from build123d import *

# Parameters (mm, degrees)
SKETCH1_W           = 140
SKETCH1_H           = 200
BOSS_EXTRUDE1_DEPTH = 30
SKETCH2_W           = 140
SKETCH2_H           = 15
CUT_EXTRUDE1_DEPTH  = 175.642491966
SKETCH3_W           = 60
SKETCH3_H           = 15
CUT_EXTRUDE3_DEPTH  = 215.00934559
SKETCH4_W           = 80
SKETCH4_H           = 140
BOSS_EXTRUDE3_DEPTH = 61
SKETCH5_W           = 100
SKETCH5_H           = 160
SKETCH5_W_2         = 70
SKETCH5_H_2         = 130
BOSS_EXTRUDE4_DEPTH = 14
SKETCH7_W           = 70
SKETCH7_H           = 130
CUT_EXTRUDE4_DEPTH  = 36
BOSS_EXTRUDE5_DEPTH = 10
BOSS_EXTRUDE6_DEPTH = 10


with BuildPart() as part:
    # Sketch1 → Boss-Extrude1 (new body)
    with BuildSketch(Plane(origin=(0, 0, 0), x_dir=(1, 0, 0), z_dir=(0, 1, 0))):
        Rectangle(SKETCH1_W, SKETCH1_H)
    extrude(amount=BOSS_EXTRUDE1_DEPTH)

    # Sketch2 → Cut-Extrude1 (cut, through all)
    with BuildSketch(Plane(origin=(70, 0, 0), x_dir=(0, 0, -1), z_dir=(1, 0, 0))):
        with Locations((0, 7.5)):
            Rectangle(SKETCH2_W, SKETCH2_H)
    extrude(amount=-CUT_EXTRUDE1_DEPTH, mode=Mode.SUBTRACT)

    # Sketch3 → Cut-Extrude3 (cut, through all)
    with BuildSketch(Plane.XY.offset(100)):
        with Locations((0, 7.5)):
            Rectangle(SKETCH3_W, SKETCH3_H)
    extrude(amount=-CUT_EXTRUDE3_DEPTH, mode=Mode.SUBTRACT)

    # Sketch4 → Boss-Extrude3 (add)
    with BuildSketch(Plane(origin=(0, 30, 0), x_dir=(1, 0, 0), z_dir=(0, 1, 0))):
        Rectangle(SKETCH4_W, SKETCH4_H)
    extrude(amount=BOSS_EXTRUDE3_DEPTH)

    # Sketch5 → Boss-Extrude4 (add)
    with BuildSketch(Plane(origin=(0, 91, 0), x_dir=(1, 0, 0), z_dir=(0, 1, 0))):
        Rectangle(SKETCH5_W, SKETCH5_H)
        Rectangle(SKETCH5_W_2, SKETCH5_H_2, mode=Mode.SUBTRACT)
    extrude(amount=BOSS_EXTRUDE4_DEPTH)

    # Sketch7 → Cut-Extrude4 (cut)
    with BuildSketch(Plane(origin=(0, 91, 0), x_dir=(1, 0, 0), z_dir=(0, 1, 0))):
        Rectangle(SKETCH7_W, SKETCH7_H)
    extrude(amount=-CUT_EXTRUDE4_DEPTH, mode=Mode.SUBTRACT)

    # Sketch9 → Boss-Extrude5 (add, symmetric)
    with BuildSketch(Plane.XY):
        Polygon((-50, 91), (-70, 30), (-39.979727261, 30), (-40, 91), align=None)
    boss_extrude5 = extrude(amount=BOSS_EXTRUDE5_DEPTH, both=True)

    # Mirror1: Boss-Extrude5 across plane
    add(boss_extrude5.mirror(Plane(origin=(0, 0, 0), x_dir=(0, 0, 1), z_dir=(1, 0, 0))))

    # Sketch10 → Boss-Extrude6 (add, symmetric)
    with BuildSketch(Plane(origin=(0, 0, 0), x_dir=(0, 0, -1), z_dir=(1, 0, 0))):
        Polygon((-70, 91), (-80, 91), (-100, 30), (-70, 30), align=None)
    boss_extrude6 = extrude(amount=BOSS_EXTRUDE6_DEPTH, both=True)

    # Mirror2: Boss-Extrude6 across plane
    add(boss_extrude6.mirror(Plane.XY))


solid = part.part
The model under review builds one solid part; all positions refer to its coordinate system, in mm. A direction names the side the tool comes from. Round coordinates to 2 decimals unless told otherwise and drop trailing zeros. Order: outer loops, then holes, each group sorted by start corner. A loop starts at its lowest first (then second) coordinate and runs counter-clockwise, first axis right, second up. Notation, with made-up numbers: (-13.75, -6) -> (15.25, -6) arc R23 cw to (15.25, 17) -> close; hole circle Ø4 at (13.5, 87). An arc over 180 degrees is marked (long way). Write item = value, one per line. Start each with the question number.
Item 1: For faces 1 (the face through (52, 54, -10)), 2 (the face through (52, 54, 10)), 3 (the face through (35, 80, 1)), 4 (the face through (-1, 98, 80)), list the 3-axis set-ups (+Z, -Z, +X, -X, +Y, -Y) from which the entire face can be reached by the end or side of a thin tool; tool diameter is ignored.
Item 2: Mouldability with a two-part tool opening along Z and no side actions: class faces 5 (the face through (30, 7, -85)), 6 (the face through (-1, 98, -80)), 7 (the face through (0, 55, -1)) as released by +Z, released by -Z, zero draft, split by the parting line, or undercut.
Item 3: Consider section B-B on x = -54. Write out the cut boundary in (y, z).
Item 4: For line 1 along Z through (x, y) = (15.5, 61.5); line 2 along Z through (x, y) = (-14.5, 96.5); line 3 along Y through (x, z) = (-44.5, 54), list the stretches that pass through material, from the lowest coordinate up.
Item 5: Consider section D-D on z = 17. Write out the cut boundary in (x, y).
Item 6: Consider section C-C on y = 63. Write out the cut boundary in (x, z).
Item 7: Consider section A-A on y = 9.5. Write out the cut boundary in (x, z).
Item 8: Clearance check with flat-ended pins moving along their axes: pin 1 Ø1.5 at (y, z) = (50, -51.5) entering from +X; pin 2 Ø24 at (x, y) = (-51, 54) entering from -Z; pin 3 Ø6 at (x, z) = (6, -18) entering from +Y. State where each tip first meets the part, or that it passes through.
Conclusion:
q1.face_1 = -Z, +X
q1.face_2 = +Z, +X
q1.face_3 = +Y
q1.face_4 = +Z, +X, -X, +Y
q2.face_5 = zero draft
q2.face_6 = released by -Z
q2.face_7 = undercut
q3.outline = (0, -100) -> (30, -100) -> (30, -10) -> (78.8, -10) -> (78.8, 10) -> (30, 10) -> (30, 100) -> (0, 100) -> (0, 70) -> (15, 70) -> (15, -70) -> (0, -70) -> close
q4.line_1 = -70 to -65, 65 to 70
q4.line_2 = -80 to -65, 65 to 80
q4.line_3 = 15 to 30, 91 to 105
q5.outline = (-70, 15) -> (70, 15) -> (70, 30) -> (40, 30) -> (40, 91) -> (50, 91) -> (50, 105) -> (35, 105) -> (35, 55) -> (-35, 55) -> (-35, 105) -> (-50, 105) -> (-50, 91) -> (-40, 91) -> (-40, 30) -> (-70, 30) -> close
q6.outline = (-59.18, -10) -> (-40, -10) -> (-40, -70) -> (-10, -70) -> (-10, -89.18) -> (10, -89.18) -> (10, -70) -> (40, -70) -> (40, -10) -> (59.18, -10) -> (59.18, 10) -> (40, 10) -> (40, 70) -> (10, 70) -> (10, 89.18) -> (-10, 89.18) -> (-10, 70) -> (-40, 70) -> (-40, 10) -> (-59.18, 10) -> close; hole (-35, -65) -> (35, -65) -> (35, 65) -> (-35, 65) -> close
q7.outline = (-70, -100) -> (-30, -100) -> (-30, -70) -> (-70, -70) -> close; (-70, 70) -> (-30, 70) -> (-30, 100) -> (-70, 100) -> close; (30, -100) -> (70, -100) -> (70, -70) -> (30, -70) -> close; (30, 70) -> (70, 70) -> (70, 100) -> (30, 100) -> close
q8.pin_1 = 40
q8.pin_2 = -70
q8.pin_3 = 55
